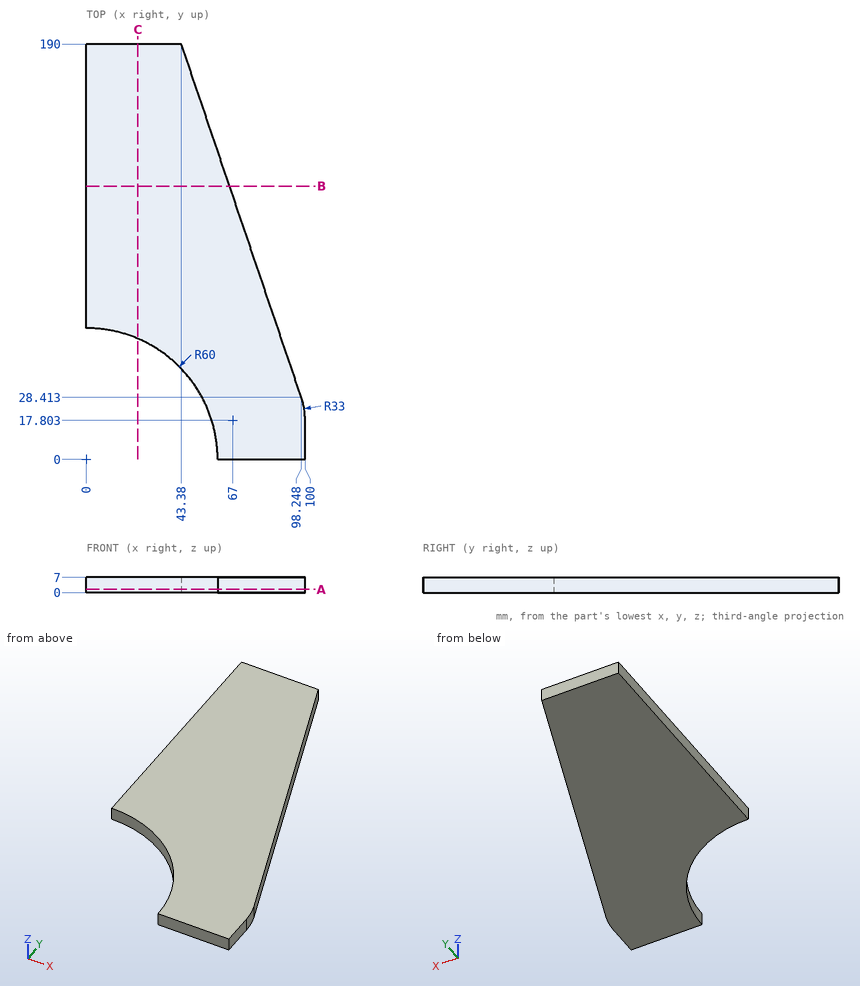
Part print with two shaded views. Sizes in mm from the minimum x, y, z corner. Give positions to 0.01 mm unless a question says otherwise; leave off trailing zeros. Write each loop counter-clockwise with the first axis right and the second up, starting at its lowest first coordinate (ties: lowest second). Pieces come first, ordered by that corner, then holes.
1) Probe L1, parallel to X at y = 10.5, z = 4; L2, parallel to X at y = 34, z = 6; L3, parallel to Y at x = 17, z = 6.25. List the from-to ranges inside material, lowest first.
Resolved:
L1: x = 59.07 to 100
L2: x = 49.44 to 96.35
L3: y = 57.54 to 190
2) Cut at C-C on x = 23.5. Write the cut outline in (y, z).
Resolved:
outline: (55.21, 0) - (190, 0) - (190, 7) - (55.21, 7) - close
3) Cut at B-B on y = 125. Write the cut outline in (x, z).
Resolved:
outline: (0, 0) - (65.45, 0) - (65.45, 7) - (0, 7) - close
4) Cut at A-A on z = 1.5. Write the cut outline in (x, y).
Resolved:
outline: (0, 60) arc R60 cw to (60, 0) - (100, 0) - (100, 17.8) arc R33 ccw to (98.25, 28.41) - (43.38, 190) - (0, 190) - close
5) Pin check, flat tips, straight feed: pin 1 (4 mm diameter, centred on x = 12.5, z = 2, fed in from -Y); pin 2 (1 mm diameter, centred on y = 128, z = 5, fed in from +X). Stop position of each tip, or through.
Resolved:
pin 1: stops at y = 58.22
pin 2: stops at x = 64.6
